The figure shows three views and two pictorial views of one solid part (mm, origin at its lowest corner). Answer the questions. A direction names the side the tool comes from. Round coordinates to 2 decimals unless told otherwise and drop trailing zeros. Order: outer loops, then holes, each group sorted by start corner. A loop starts at its lowest first (then second) coordinate and runs counter-clockwise, first axis right, second up. Notation, with made-up numbers: (56, 49) - (100, 49) arc R15 cw to (100, 57) - close; hole circle Ø1 at (32.5, -36.75). An arc over 180 degrees is marked (long way). Write item = value, one per line.
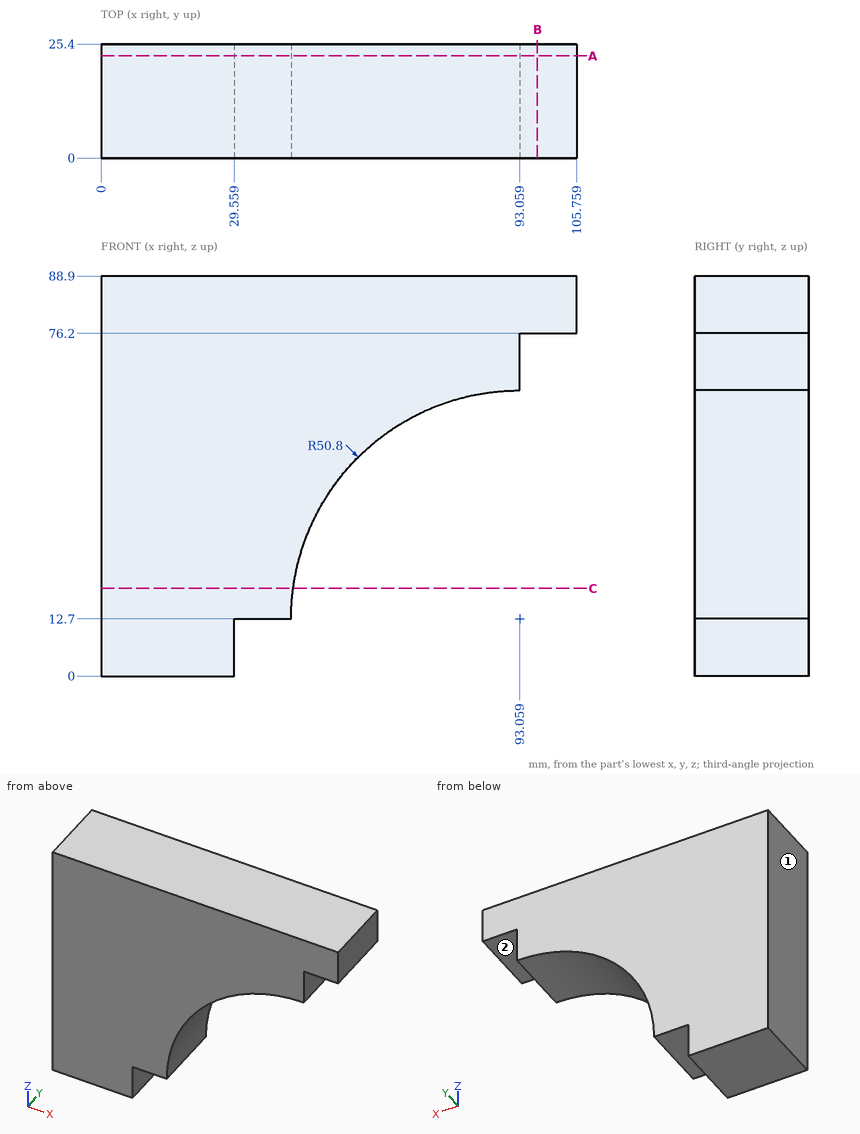
Q1. Section B-B on x = 97 is taken. Determine the outline of the cut face in (y, z).
Model answer:
outline = (0, 76.2) - (25.4, 76.2) - (25.4, 88.9) - (0, 88.9) - close
Q2. Section C-C on z = 19.5 is taken. Determine the outline of the cut face in (x, y) (1 decimal).
Model answer:
outline = (0, 0) - (42.7, 0) - (42.7, 25.4) - (0, 25.4) - close
Q3. For the marked faces 1 and 2, determine the directions among +Z, -Z, +X, -X, +Y, -Y from which every point of the face is accessible in a straight line to the end or side of a thin tool.
Model answer:
face_1 = +Z, -Z, -X, +Y, -Y
face_2 = -Z, +X, +Y, -Y
Q4. Find the intervals of material crossed by line 1 (Z direction, x = 41.5, y = 13.5); line 2 (X direction, y = 13.25, z = 8.5); line 3 (Z direction, x = 100, y = 8), in increasing order. Write a range as from..to.
Model answer:
line_1 = 12.7..88.9
line_2 = 0..29.56
line_3 = 76.2..88.9
Q5. Flat-ended cylindrical pins translate along their axes: P1, Ø6.5, axis at x = 35, y = 8.5, coming from the -Z side; P2, Ø14, axis at x = 99.5, y = 9.5, coming from the -Z side; P3, Ø6.5, axis at y = 9.5, z = 70, coming from the +X side. Find the tip coordinate at first contact, or state that the pin passes through.
Model answer:
P1 = 12.7
P2 = 63.5
P3 = 93.06
Q6. Section A-A on y = 22.75 is taken. Determine the outline of the cut face in (x, z).
Model answer:
outline = (0, 0) - (29.56, 0) - (29.56, 12.7) - (42.26, 12.7) arc R50.8 cw to (93.06, 63.5) - (93.06, 76.2) - (105.76, 76.2) - (105.76, 88.9) - (0, 88.9) - close
